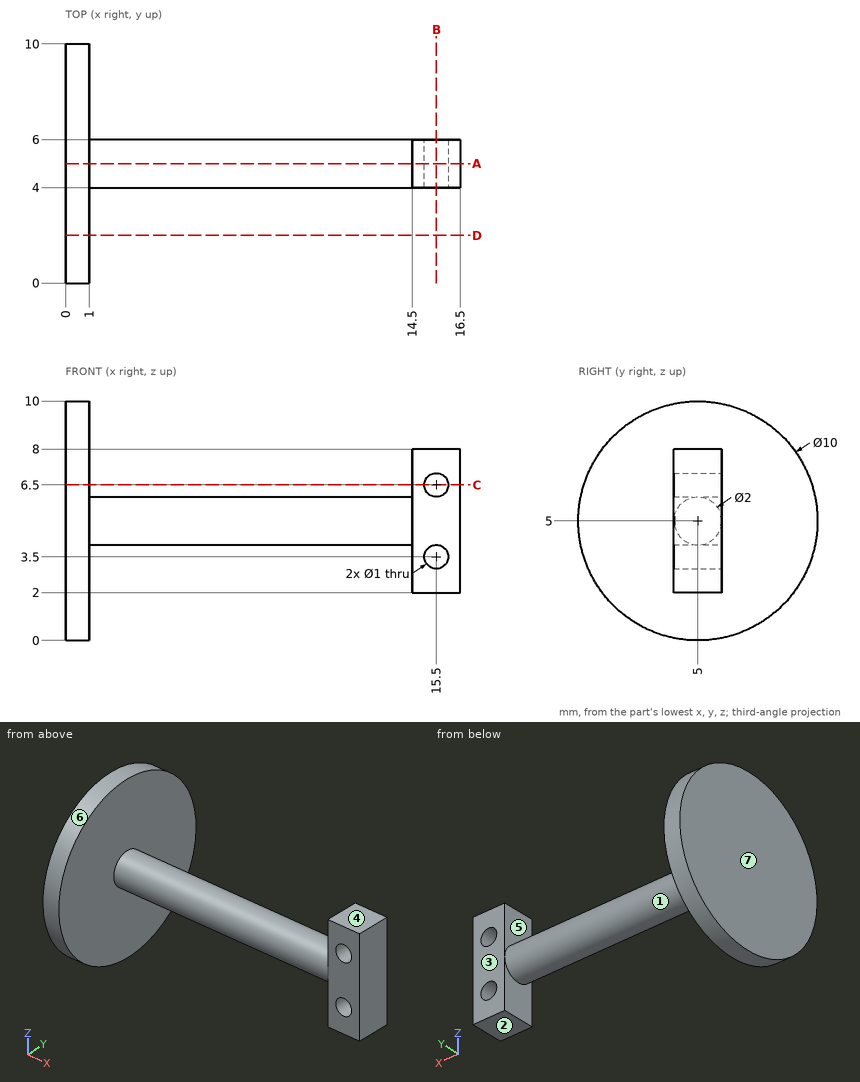
Geometry check sheet. Reference: drawing and pictorial views, mm from the part's lowest x, y, z. A direction names the side the tool comes from. Give positions to 0.01 mm unless a question says otherwise; leave off trailing zeros. Order: outer loops, then holes, each group sorted by start corner. A loop starts at its lowest first (then second) coordinate and runs counter-clockwise, first axis right, second up. Notation, with made-up numbers: M -17,-2.75 L 26,-2.75 A19 ccw 26,3.25 Z; hole C 2.5,19 d6. An arc over 180 degrees is marked long. Return JSON: item names as keys, results as strings. Group by question number.
1) Mould release check, pull along X, two halves, no side actions. Record for the marked faces 5, 6 and 7: pulls with the +X half, pulls with the -X half, needs draft (parallel to the pull), parting line crosses it, or undercut.
2) Section check B-B on x = 15.5. Record the cut outline in (y, z).
3) Scan lines: line 1 (X direction, y = 4.85, z = 6.5); line 2 (Z direction, x = 15.5, y = 5.5); line 3 (Z direction, x = 12.5, y = 5). Record each from-to range of solid material in increasing order.
4) Section check C-C on z = 6.5. Record the cut outline in (x, y).
5) Section check A-A on y = 5. Record the cut outline in (x, z).
6) Go/stop test with flat-tipped pins: pin 1 Ø5 at (x, y) = (5.5, 5) entering from -Z; pin 2 Ø0.6 at (x, z) = (15, 6) entering from +Y; pin 3 Ø0.6 at (x, y) = (15.5, 5.5) entering from -Z. Record where each tip stops, or that it passes through.
7) Access from +Z, -Z, +X, -X, +Y, -Y to the whole of each face (thin tool, end or side, straight path). Record for the marked faces 1, 2, 3 and 4.
8) Section check D-D on y = 2. Record the cut outline in (x, z).
Answer block:
{
 "1": {"face 5": "undercut", "face 6": "needs draft", "face 7": "pulls with the -X half"},
 "2": {"outline": "M 4,2 L 6,2 L 6,3 L 4,3 Z; M 4,4 L 6,4 L 6,6 L 4,6 Z; M 4,7 L 6,7 L 6,8 L 4,8 Z"},
 "3": {"line 1": "x = 0 to 1, 14.5 to 15, 16 to 16.5", "line 2": "z = 2 to 3, 4 to 6, 7 to 8", "line 3": "z = 4 to 6"},
 "4": {"outline": "M 0,0.23 L 1,0.23 L 1,9.77 L 0,9.77 Z; M 14.5,4 L 15,4 L 15,6 L 14.5,6 Z; M 16,4 L 16.5,4 L 16.5,6 L 16,6 Z"},
 "5": {"outline": "M 0,0 L 1,0 L 1,4 L 14.5,4 L 14.5,2 L 16.5,2 L 16.5,8 L 14.5,8 L 14.5,6 L 1,6 L 1,10 L 0,10 Z; hole C 15.5,3.5 d1; hole C 15.5,6.5 d1"},
 "6": {"pin 1": "stops at z = 4", "pin 2": "stops at y = 6", "pin 3": "stops at z = 2"},
 "7": {"face 1": "none", "face 2": "-Z, +X, +Y, -Y", "face 3": "+Z, -Z, +X, +Y", "face 4": "+Z, +X, +Y, -Y"},
 "8": {"outline": "M 0,1 L 1,1 L 1,9 L 0,9 Z"}
}
